```python
from build123d import *

# Parameters (mm, degrees)
F0_W     = 76.2
F0_H     = 76.2
F1_DEPTH = 25.4
F2_R     = 26.590625
F3_DEPTH = 12.7
F4_R     = 1.27
F6_DEPTH = 25.4


with BuildPart() as f1:
    # F0 (on Top) → F1 (new body)
    with BuildSketch(Plane.XY):
        Rectangle(F0_W, F0_H)
    extrude(amount=F1_DEPTH)

    # F2 (on face) → F3 (cut)
    with BuildSketch(Plane(origin=(0, 0, 0), x_dir=(1, 0, 0), z_dir=(0, 0, -1))):
        Circle(F2_R)
    extrude(amount=-F3_DEPTH, mode=Mode.SUBTRACT)

    # F4
    f4_edges = [f1.edges().sort_by_distance(p)[0] for p in [
        (0, -38.1, 25.4),
        (0, 38.1, 25.4),
        (38.1, 0, 25.4),
        (38.1, -38.1, 12.7),
        (38.1, 38.1, 12.7),
        (-38.1, 38.1, 12.7),
        (-38.1, -38.1, 12.7),
        (-38.1, 0, 25.4),
        (0, -38.1, 0),
        (-38.1, 0, 0),
        (0, 38.1, 0),
        (38.1, 0, 0),
    ]]
    fillet(f4_edges, radius=F4_R)

    # F5 (on face) → F6 (cut)
    with BuildSketch(Plane.XY.offset(25.4)):
        Polygon((1.5875, -2.749631), (3.175, 0), (1.5875, 2.749631), (-1.5875, 2.749631), (-3.175, 0), (-1.5875, -2.749631), align=None)
        Polygon((-3.175, 6.769261), (-1.5875, 4.019631), (1.5875, 4.019631), (3.175, 6.769261), (1.5875, 9.518892), (-1.5875, 9.518892), align=None)
        Polygon((-9.037352, 3.384631), (-7.449852, 0.635), (-4.274852, 0.635), (-2.687352, 3.384631), (-4.274852, 6.134261), (-7.449852, 6.134261), align=None)
        Polygon((-7.449852, -6.134261), (-4.274852, -6.134261), (-2.687352, -3.384631), (-4.274852, -0.635), (-7.449852, -0.635), (-9.037352, -3.384631), align=None)
        Polygon((1.5875, -9.518892), (3.175, -6.769261), (1.5875, -4.019631), (-1.5875, -4.019631), (-3.175, -6.769261), (-1.5875, -9.518892), align=None)
        Polygon((9.037352, -3.384631), (7.449852, -0.635), (4.274852, -0.635), (2.687352, -3.384631), (4.274852, -6.134261), (7.449852, -6.134261), align=None)
        Polygon((7.449852, 6.134261), (4.274852, 6.134261), (2.687352, 3.384631), (4.274852, 0.635), (7.449852, 0.635), (9.037352, 3.384631), align=None)
        Polygon((4.274852, 7.404261), (7.449852, 7.404261), (9.037352, 10.153892), (7.449852, 12.903523), (4.274852, 12.903523), (2.687352, 10.153892), align=None)
        Polygon((-7.449852, 12.903523), (-9.037352, 10.153892), (-7.449852, 7.404261), (-4.274852, 7.404261), (-2.687352, 10.153892), (-4.274852, 12.903523), align=None)
        Polygon((-14.899705, 0), (-13.312205, -2.749631), (-10.137205, -2.749631), (-8.549705, 0), (-10.137205, 2.749631), (-13.312205, 2.749631), align=None)
        Polygon((-7.449852, -12.903523), (-4.274852, -12.903523), (-2.687352, -10.153892), (-4.274852, -7.404261), (-7.449852, -7.404261), (-9.037352, -10.153892), align=None)
        Polygon((7.449852, -12.903523), (9.037352, -10.153892), (7.449852, -7.404261), (4.274852, -7.404261), (2.687352, -10.153892), (4.274852, -12.903523), align=None)
        Polygon((14.899705, 0), (13.312205, 2.749631), (10.137205, 2.749631), (8.549705, 0), (10.137205, -2.749631), (13.312205, -2.749631), align=None)
        Polygon((-1.5875, 10.788892), (1.5875, 10.788892), (3.175, 13.538523), (1.5875, 16.288153), (-1.5875, 16.288153), (-3.175, 13.538523), align=None)
        Polygon((-13.312205, 9.518892), (-14.899705, 6.769261), (-13.312205, 4.019631), (-10.137205, 4.019631), (-8.549705, 6.769261), (-10.137205, 9.518892), align=None)
        Polygon((-14.899705, -6.769261), (-13.312205, -9.518892), (-10.137205, -9.518892), (-8.549705, -6.769261), (-10.137205, -4.019631), (-13.312205, -4.019631), align=None)
        Polygon((-1.5875, -16.288153), (1.5875, -16.288153), (3.175, -13.538523), (1.5875, -10.788892), (-1.5875, -10.788892), (-3.175, -13.538523), align=None)
        Polygon((13.312205, -9.518892), (14.899705, -6.769261), (13.312205, -4.019631), (10.137205, -4.019631), (8.549705, -6.769261), (10.137205, -9.518892), align=None)
        Polygon((14.899705, 6.769261), (13.312205, 9.518892), (10.137205, 9.518892), (8.549705, 6.769261), (10.137205, 4.019631), (13.312205, 4.019631), align=None)
    extrude(amount=-F6_DEPTH, mode=Mode.SUBTRACT)


solid = f1.part
```
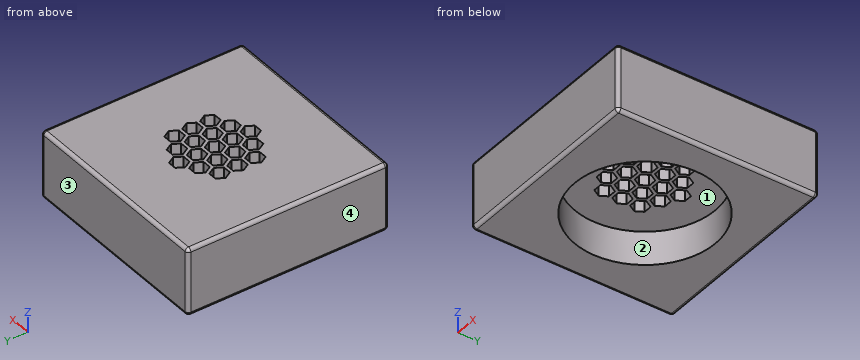
Read the model definition and answer for the solid it produces. Units are mm, in the model's axes. Face numbers are marked on the shaded views. Give positions to 0.01 mm unless a question says otherwise; leave off trailing zeros. Order: outer loops, then holes, each group sorted by start corner. A loop starts at its lowest first (then second) coordinate and runs counter-clockwise, first axis right, second up. Notation, with made-up numbers: (-28.75, 29.25) -> (27.25, 29.25) arc R25 ccw to (27.25, 44.25) -> close; hole circle Ø9 at (-33.5, -25). An arc over 180 degrees is marked (long way). Write item = value, one per line.
1. A cutting plane is placed at D-D, the plane y = -24. Write down the section's boundary in (x, z), and give its area (3 significant figures).
Numbers:
outline = (-38.1, 1.27) arc R1.27 ccw to (-36.83, 0) -> (-11.45, 0) -> (-11.45, 12.7) -> (11.45, 12.7) -> (11.45, 0) -> (36.83, 0) arc R1.27 ccw to (38.1, 1.27) -> (38.1, 24.13) arc R1.27 ccw to (36.83, 25.4) -> (-36.83, 25.4) arc R1.27 ccw to (-38.1, 24.13) -> close
area = 1,640 mm²
2. Straight lines are drawn through the part: line 1 along Y through (x, z) = (-4.5, 17) (3 decimals); line 2 along Y through (x, z) = (0, 5.5). For each, find the intervals that lie inside material, in ascending order.
Numbers:
line_1 = -38.1 to -12.904, -7.404 to -6.134, -0.635 to 0.635, 6.134 to 7.404, 12.904 to 38.1
line_2 = -38.1 to -26.59, 26.59 to 38.1
3. The mould has two halves that part along Y. Classify the marked faces 1, 2, 3 and 4: +Y half, -Y half, draft (parallel to the pull), parting line (faces both ways), or undercut.
Numbers:
face_1 = undercut
face_2 = undercut
face_3 = +Y half
face_4 = draft
4. Given pin 1 (10 mm diameter, centred on x = -4.5, y = 1.5, fed in from -Z), flat-ended and moving along its own axis, determine where the tip first touches the part or whether it passes through.
Numbers:
pin_1 = 12.7
5. A cutting plane is placed at B-B, the plane z = 5.75. Write down the section's boundary in (x, y).
Numbers:
outline = (-38.1, -36.83) arc R1.27 ccw to (-36.83, -38.1) -> (36.83, -38.1) arc R1.27 ccw to (38.1, -36.83) -> (38.1, 36.83) arc R1.27 ccw to (36.83, 38.1) -> (-36.83, 38.1) arc R1.27 ccw to (-38.1, 36.83) -> close; hole circle Ø53.18 at (0, 0)
6. A cutting plane is placed at A-A, the plane x = 0. Count the separate pieces of the cut face and the enclosed holes in it, and give its area (3 significant figures).
Numbers:
separate_pieces = 6
enclosed_holes = 0
area = 909 mm²
